The model under review builds one solid part; all positions refer to its coordinate system, in mm. Face numbers are marked on the shaded views. Give positions to 0.01 mm unless a question says otherwise; leave off trailing zeros. Order: outer loops, then holes, each group sorted by start corner. A loop starts at its lowest first (then second) coordinate and runs counter-clockwise, first axis right, second up. Notation, with made-up numbers: (-19.5, 19) - (16.5, 19) arc R27 ccw to (16.5, 39) - close; hole circle Ø2 at (31.25, 26). An arc over 180 degrees is marked (long way). Use CSV: the item, a comma, the result in double quotes. Start each with the question number.
1. Take a section at A-A, the plane y = -11.45. State the section outline as (x, z) points.
2. For pin 1 (8 mm diameter, centred on x = 25, y = 26, fed in from -Z); pin 2 (10 mm diameter, centred on x = 0, y = -3.33, fed in from +Z); pin 3 (3 mm diameter, centred on x = 25, z = 9.99, fed in from +Y); pin 4 (2.5 mm diameter, centred on x = 1, y = -57, fed in from +Z), all flat-tipped, find the tip position at first contact; note any pin that passes through.
3. Draft analysis for pull direction X (two halves, no side actions). For the marked faces 1, 2 and 3, state which applies: released by +X, released by -X, zero draft, split by the parting line, or undercut.
4. Take a section at B-B, the plane y = 15.5. State the section outline as (x, z) points.
5. To check wall thickness, follow line 1 (Y direction, x = -25, z = 2.05); line 2 (Y direction, x = 0, z = 2.1); line 3 (Y direction, x = 0, z = 3). State the ranges of each line that lie inside material, in increasing order. Write a range as [from, to].
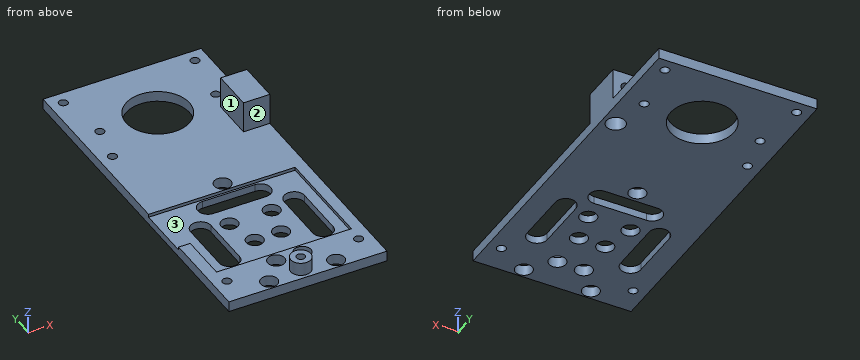
```python
from build123d import *

# Parameters (mm, degrees)
SKETCH_R        = 3.2
SKETCH_R_2      = 1.7
SKETCH_R_3      = 3.6
SKETCH_R_4      = 12
PAD_DEPTH       = 4
POCKET_DEPTH    = 1.2
SKETCH005_R     = 3.8
PAD002_DEPTH    = 5
SKETCH007_R     = 2
POCKET004_DEPTH = 12
SKETCH011_R     = 2
POCKET006_DEPTH = 10
SKETCH012_R     = 1.6
POCKET007_DEPTH = 8
SKETCH013_W     = 10
SKETCH013_H     = 16
PAD003_DEPTH    = 12
SKETCH014_R     = 3.6
POCKET008_DEPTH = 10
SKETCH015_R     = 2
POCKET009_DEPTH = 10
SKETCH016_R     = 1.7
POCKET010_DEPTH = 5


with BuildPart() as part:
    # Sketch → Pad (new body)
    with BuildSketch(Plane.XY):
        Polygon((30, -63), (-30, -63), (-30, 67), (0, 67), (30, 67), (30, -2), (30, -22), (30, -41), align=None)
        with Locations((-12.71, -59.3)):
            Circle(SKETCH_R, mode=Mode.SUBTRACT)
        with Locations((12.71, -59.3)):
            Circle(SKETCH_R, mode=Mode.SUBTRACT)
        with Locations((0, -3.33)):
            Circle(SKETCH_R, mode=Mode.SUBTRACT)
        with Locations((-8, -22.917882)):
            Circle(SKETCH_R, mode=Mode.SUBTRACT)
        with Locations((8, -22.917882)):
            Circle(SKETCH_R, mode=Mode.SUBTRACT)
        with Locations((-5, -35)):
            Circle(SKETCH_R, mode=Mode.SUBTRACT)
        with Locations((5, -35)):
            Circle(SKETCH_R, mode=Mode.SUBTRACT)
        with Locations((-5, -50)):
            Circle(SKETCH_R, mode=Mode.SUBTRACT)
        with Locations((5, -50)):
            Circle(SKETCH_R, mode=Mode.SUBTRACT)
        with Locations((-25, -52.39)):
            Circle(SKETCH_R_2, mode=Mode.SUBTRACT)
        with Locations((25, -52.39)):
            Circle(SKETCH_R_2, mode=Mode.SUBTRACT)
        with Locations((-25, 27.61)):
            Circle(SKETCH_R_2, mode=Mode.SUBTRACT)
        with Locations((25, 27.61)):
            Circle(SKETCH_R_3, mode=Mode.SUBTRACT)
        with Locations((0, 42)):
            Circle(SKETCH_R_4, mode=Mode.SUBTRACT)
        with Locations((-22, 42)):
            Circle(SKETCH_R_2, mode=Mode.SUBTRACT)
        with Locations((22, 42)):
            Circle(SKETCH_R_2, mode=Mode.SUBTRACT)
        with BuildLine():
            ThreePointArc((-21.6, -40.75), (-17.75, -44.6), (-13.9, -40.75))
            Line((-13.9, -40.75), (-13.9, -20.75))
            ThreePointArc((-13.9, -20.75), (-17.75, -16.9), (-21.6, -20.75))
            Line((-21.6, -40.75), (-21.6, -20.75))
        make_face(mode=Mode.SUBTRACT)
        with BuildLine():
            ThreePointArc((13.9, -40.75), (17.75, -44.6), (21.6, -40.75))
            Line((21.6, -40.75), (21.6, -20.75))
            ThreePointArc((21.6, -20.75), (17.75, -16.9), (13.9, -20.75))
            Line((13.9, -40.75), (13.9, -20.75))
        make_face(mode=Mode.SUBTRACT)
        with BuildLine():
            ThreePointArc((-10, -7.6), (-13.85, -11.45), (-10, -15.3))
            Line((-10, -15.3), (10, -15.3))
            ThreePointArc((10, -15.3), (13.85, -11.45), (10, -7.6))
            Line((-10, -7.6), (10, -7.6))
        make_face(mode=Mode.SUBTRACT)
    extrude(amount=PAD_DEPTH)

    # Sketch001 (on Face38 of Pad) → Pocket (cut)
    with BuildSketch(Plane.XY.offset(4)):
        Polygon((25.61, -46.249557), (-25.61, -46.249557), (-25.61, -27.85), (-30, -27.85), (-30, -6.85), (-25.701572, -6.85), (25.61, -6.85), align=None)
    extrude(amount=-POCKET_DEPTH, mode=Mode.SUBTRACT)

    # Sketch005 → Pad002 (join)
    with BuildSketch(Plane.XY.offset(4)):
        with Locations((0, -58)):
            Circle(SKETCH005_R)
    extrude(amount=PAD002_DEPTH)

    # Sketch007 → Pocket004 (cut)
    with BuildSketch(Plane(origin=(25.61, 0, 0), x_dir=(0, -1, 0), z_dir=(-1, 0, 0))):
        with Locations((-25, 10.599272)):
            Circle(SKETCH007_R)
    extrude(amount=-POCKET004_DEPTH, mode=Mode.SUBTRACT)

    # Sketch011 → Pocket006 (cut)
    with BuildSketch(Plane.YZ.offset(30)):
        with Locations((-25, -5.497445)):
            Circle(SKETCH011_R)
    extrude(amount=-POCKET006_DEPTH, mode=Mode.SUBTRACT)

    # Sketch012 (on Face47 of Pocket006) → Pocket007 (cut)
    with BuildSketch(Plane.XY.offset(9)):
        with Locations((0, -58)):
            Circle(SKETCH012_R)
    extrude(amount=-POCKET007_DEPTH, mode=Mode.SUBTRACT)

    # Sketch013 (on Face5 of Pocket007) → Pad003 (join)
    with BuildSketch(Plane.XY.offset(4)):
        with Locations((25, 26.940226)):
            Rectangle(SKETCH013_W, SKETCH013_H)
    extrude(amount=PAD003_DEPTH)

    # Sketch014 (on Face51 of Pad003) → Pocket008 (cut)
    with BuildSketch(Plane(origin=(0, 0, 4), x_dir=(1, 0, 0), z_dir=(0, 0, -1))):
        with Locations((25, -27.61)):
            Circle(SKETCH014_R)
    extrude(amount=-POCKET008_DEPTH, mode=Mode.SUBTRACT)

    # Sketch015 (on Face41 of Pocket008) → Pocket009 (cut)
    with BuildSketch(Plane(origin=(0, 34.940226, 0), x_dir=(-1, 0, 0), z_dir=(0, 1, 0))):
        with Locations((-25, 9.985852)):
            Circle(SKETCH015_R)
    extrude(amount=-POCKET009_DEPTH, mode=Mode.SUBTRACT)

    # Sketch016 (on Face5 of Pocket009) → Pocket010 (cut)
    with BuildSketch(Plane.XY.offset(4)):
        with Locations((-25, 62)):
            Circle(SKETCH016_R)
        with Locations((25, 62)):
            Circle(SKETCH016_R)
    extrude(amount=-POCKET010_DEPTH, mode=Mode.SUBTRACT)


solid = part.part
```
Determined:
1,outline,"(-30, 0) - (-13.85, 0) - (-13.85, 2.8) - (-30, 2.8) - close; (13.85, 0) - (30, 0) - (30, 4) - (25.61, 4) - (25.61, 2.8) - (13.85, 2.8) - close"
2,pin 1,"stops at z = 0"
2,pin 2,"stops at z = 4"
2,pin 3,"stops at y = 24.34"
2,pin 4,"stops at z = 9"
3,face 1,"released by -X"
3,face 2,"zero draft"
3,face 3,"undercut"
4,outline,"(-30, 0) - (30, 0) - (30, 4) - (-30, 4) - close"
5,line 1,"y = [-63, -54.09], [-50.69, 25.91], [29.31, 60.3], [63.7, 67]"
5,line 2,"y = [-63, -59.6], [-56.4, -15.3], [-7.6, -6.53], [-0.13, 30], [54, 67]"
5,line 3,"y = [-63, -59.6], [-56.4, -46.25], [-6.85, -6.53], [-0.13, 30], [54, 67]"
